from build123d import *
from build123d.topology import SkipClean

# Parameters (mm, degrees)
REVOLVE1_ANGLE                  = 180
SKETCH3_R                       = 26
CUT_EXTRUDE1_DEPTH              = 10
SKETCH6_R                       = 8
BOSS_EXTRUDE2_DEPTH             = 35
BOSS_EXTRUDE2_DIRECTION_2_REACH = 133.642
CUT_EXTRUDE8_DEPTH              = 35
CUT_EXTRUDE8_DEPTH_BACK         = 10
SKETCH6_6_R                     = 6.5
SKETCH7_W                       = 164.845441074
SKETCH7_H                       = 52.750628287
CUT_EXTRUDE9_DEPTH              = 109.712015004


with BuildPart() as part:
    # Sketch1 → Revolve1 (revolve)
    with BuildSketch(Plane.XY):
        Polygon((26, 40), (61, 0), (65.013813376, -0.015786716), (30, 40), align=None)
    revolve1 = revolve(axis=Axis((0, 40, 0), (0, -1, 0)), revolution_arc=REVOLVE1_ANGLE)

    # Sketch3 → Cut-Extrude1 (cut)
    with BuildSketch(Plane(origin=(0, 32.212389381, 36.814159292), x_dir=(1, 0, 0), z_dir=(0, 0.6585046078685183, 0.7525766947068778))):
        with Locations((0, -20.352106134)):
            Circle(SKETCH3_R)
    extrude(amount=-CUT_EXTRUDE1_DEPTH, mode=Mode.SUBTRACT)

    # Mirror1: Revolve1 across plane
    add(revolve1.mirror(Plane.XY))

    # Sketch6 → Boss-Extrude2 (add)
    with BuildSketch(Plane(origin=(9.948450871, 26.808829171, -41.542274476), x_dir=(-1, 0, 0), z_dir=(0, 0.15372802298718932, -0.9881131994606945))):
        with Locations(Location((0, 0, 0), (0, 0, 90))):
            Circle(SKETCH6_R)
    extrude(amount=BOSS_EXTRUDE2_DEPTH)

    # Boss-Extrude2 direction 2: up to this cone (the profile starts outside it)
    with SkipClean():  # the faces are left unmerged after this step: merging them gives an invalid solid
        boss_extrude2_direction_2_end = Plane(origin=(0, 26.808829, 0), z_dir=(0, -1, 0)).offset(-47.476884286) * Cone(1e-06, 195.266014922, 223.161158911, align=(Align.CENTER, Align.CENTER, Align.MIN), mode=Mode.PRIVATE)
        # Sketch6 → Boss-Extrude2 direction 2 (add, up to the surface)
        with BuildSketch(Plane(origin=(9.948450871, 26.808829171, -41.542274476), x_dir=(-1, 0, 0), z_dir=(0, 0.15372802298718932, -0.9881131994606945)), mode=Mode.PRIVATE) as boss_extrude2_direction_2_sk1:
            with Locations(Location((0, 0, 0), (0, 0, 90))):
                Circle(SKETCH6_R)
        boss_extrude2_direction_2_tool1 = extrude(boss_extrude2_direction_2_sk1.sketch, amount=-BOSS_EXTRUDE2_DIRECTION_2_REACH, mode=Mode.PRIVATE) - boss_extrude2_direction_2_end
        add(boss_extrude2_direction_2_tool1.solids().sort_by_distance((9.948451, 26.808829, -41.542274))[0])

    # Sketch6<6> → Cut-Extrude8 (cut, two sides: drawn at the far end of the back side and taken through both)
    with BuildSketch(Plane(origin=(9.948450871, 26.808829171, -41.542274476), x_dir=(-1, 0, 0), z_dir=(0, 0.15372802298718932, -0.9881131994606945)).offset(-CUT_EXTRUDE8_DEPTH_BACK)):
        with Locations(Location((0, 0, 0), (0, 0, 90))):
            Circle(SKETCH6_6_R)
    extrude(amount=CUT_EXTRUDE8_DEPTH + CUT_EXTRUDE8_DEPTH_BACK, mode=Mode.SUBTRACT)

    # Sketch7 → Cut-Extrude9 (cut, through all)
    with BuildSketch(Plane.XY):
        with Locations((11.116613387, 15.529637373)):
            Rectangle(SKETCH7_W, SKETCH7_H)
    extrude(amount=CUT_EXTRUDE9_DEPTH, mode=Mode.SUBTRACT)


solid = part.part
Input: part model. Units: mm. Frame: model coordinates. Give positions to 0.01 mm unless a question says otherwise; leave off trailing zeros. Write each loop counter-clockwise with the first axis right and the second up, starting at its lowest first coordinate (ties: lowest second). Pieces come first, ordered by that corner, then holes. Notation, with made-up numbers: M 61,-2.75 L 114,-2.75 A25 cw 114,11.25 Z; hole C 38,32.5 d5. An arc over 180 degrees is marked long. Write item = value, one per line. Start each with the question number.
1) First-contact query: pin 1 Ø12 at (x, z) = (35.5, -16.5) entering from -Y; pin 2 Ø1 at (x, y) = (43, 26.5) entering from -Z; pin 3 Ø4 at (x, z) = (-35, -11) entering from +Y; pin 4 Ø8 at (x, y) = (43, 8.5) entering from -Z. Flat tips, straight axial feed; report the tip coordinate or a pass-through.
2) Material intervals for line 1 along X through (y, z) = (28.5, -73); line 2 along X through (y, z) = (9.5, -29.5); line 3 along Z through (x, y) = (-10, 15), sorted ascending. Write a range as [from, to].
3) Cut plane A-A on x = 0. Return the cut outline in (y, z), then the cut area to 3 significant figures.
4) Cut plane B-B on y = 4. Return the cut outline in (x, z), then the cut area to 3 significant figures.
5) Draft query along Y for faces 1 (the flat face through (-46, 20, 0)), 2 (the conical face through (1.3, 0, -61.2)), 3 (the flat face through (-0.1, 40, -26.2)), 4 (the cylindrical face through (11.901, 34.846, -52.875)). Return one class per face: +Y half, -Y half, draft (parallel to the pull), parting line (faces both ways), or undercut.
6) Cut plane C-C on z = -51.5. Count the separate pieces of the cut face and the enclosed holes in it, then the cut area to 3 significant figures.
Solved:
q1.pin_1 = 18.12
q1.pin_2 = through
q1.pin_3 = 34.64
q1.pin_4 = -44.67
q2.line_1 = [2.6, 4.27], [15.63, 17.3]
q2.line_2 = [-48.41, -43.65], [43.65, 48.41]
q2.line_3 = [-50.9, -46.82]
q3.outline = M -0.02,-65.01 L 40,-30 L 40,-26 L 0,-61 Z
q3.area = 160 mm2
q4.outline = M -61.5,0 A61.5 ccw 61.5,0 L 57.5,0 A57.5 cw -57.5,0 Z
q4.area = 748 mm2
q5.face_1 = draft
q5.face_2 = -Y half
q5.face_3 = +Y half
q5.face_4 = undercut
q6.separate_pieces = 2
q6.enclosed_holes = 1
q6.area = 401 mm2
